```python
from build123d import *

# Parameters (mm, degrees)
F0_R     = 24.13
F1_DEPTH = 17.78
F2_R     = 39.733027
F2_R_2   = 24.13
F3_DEPTH = 25.4
F4_R     = 27.837104
F5_DEPTH = 19.05
F6_R     = 15.212569
F7_DEPTH = 12.7


with BuildPart() as f1:
    # F0 (on Top) → F1 (new body)
    with BuildSketch(Plane.XY):
        with Locations((-89.226432, 10.949461)):
            Circle(F0_R)
    extrude(amount=F1_DEPTH)

    # F2 (on face) → F3 (join)
    with BuildSketch(Plane.XY.offset(17.78)):
        with Locations((-89.226432, 10.949461)):
            Circle(F2_R)
        with Locations((-89.226432, 10.949461)):
            Circle(F2_R_2, mode=Mode.SUBTRACT)
        with Locations((-89.226432, 10.949461)):
            Circle(F2_R_2)
    extrude(amount=F3_DEPTH)

    # F4 (on face) → F5 (join)
    with BuildSketch(Plane.XY.offset(43.18)):
        with Locations((-89.226432, 10.949461)):
            Circle(F4_R)
    extrude(amount=F5_DEPTH)

    # F6 (on face) → F7 (join)
    with BuildSketch(Plane.XY.offset(62.23)):
        with Locations((-89.226432, 10.949461)):
            Circle(F6_R)
    extrude(amount=F7_DEPTH)


solid = f1.part
```
The model under review builds one solid part; all positions refer to its coordinate system, in mm. A direction names the side the tool comes from. Give positions to 0.01 mm unless a question says otherwise; leave off trailing zeros. Order: outer loops, then holes, each group sorted by start corner. A loop starts at its lowest first (then second) coordinate and runs counter-clockwise, first axis right, second up. Notation, with made-up numbers: (20, -7.5) - (36, -7.5) arc R16 ccw to (36, -0.5) - close; hole circle Ø2 at (75, 73). An arc over 180 degrees is marked (long way). Use CSV: the item, a comma, the result in double quotes. Start each with the question number.
Q1. We need section A-A, the plane x = -93. Write out the cut boundary in (y, z), and give its area (3 significant figures).
Q2. Clearance check with flat-ended pins moving along their axes: pin 1 Ø10 at (y, z) = (36.5, 51) entering from +X; pin 2 Ø1.5 at (x, y) = (-84, -8) entering from +Z; pin 3 Ø8 at (y, z) = (-9, 62.5) entering from +X. State where each tip first meets the part, or that it passes through.
Q3. Tool access review of faces 3 (the flat face through (-90, -15, 17.78)), 4 (the cylindrical face through (-74.716, 15.519, 68.491)), 5 (the cylindrical face through (-51.328, 22.884, 30.302)): name each direction out of +Z, -Z, +X, -X, +Y, -Y from which nothing blocks a thin tool from reaching the whole face with its end or side.
Q4. We need section C-C, the plane z = 66.5. Write out the cut boundary in (x, y).
Q5. To check wall thickness, follow line 1 along Z through (x, y) = (-90, -22); line 2 along Z through (x, y) = (-92, -7.5); line 3 along Y through (x, z) = (-88, 58). State the ranges of each line that lie inside material, in increasing order. Write a range as [from, to].
Q6. The part is to be moulded in two halves that separate along Y. For faces 1 (the flat face through (-89, 11, 74.93)), 2 (the cylindrical face through (-111.317, -5.989, 52.572)), say which applies: +Y half, -Y half, draft (parallel to the pull), parting line (faces both ways), or undercut.
Q7. We need section B-B, the plane y = 28. Write out the cut boundary in (x, z), and give its area (3 significant figures).
Q8. We need section D-D, the plane y = -6. Write out the cut boundary in (x, z).
Outcome:
1,outline,"(-28.6, 17.78) - (-12.88, 17.78) - (-12.88, 0) - (34.78, 0) - (34.78, 17.78) - (50.5, 17.78) - (50.5, 43.18) - (38.53, 43.18) - (38.53, 62.23) - (25.69, 62.23) - (25.69, 74.93) - (-3.79, 74.93) - (-3.79, 62.23) - (-16.63, 62.23) - (-16.63, 43.18) - (-28.6, 43.18) - close"
1,area,"4,280 mm^2"
2,pin 1,"stops at x = -70.45"
2,pin 2,"stops at z = 62.23"
2,pin 3,"stops at x = -66.42"
3,face 3,"-Z"
3,face 4,"+Z"
3,face 5,"+Z, -Z"
4,outline,"circle Ø30.43 at (-89.23, 10.95)"
5,line 1,"z = [17.78, 43.18]"
5,line 2,"z = [0, 62.23]"
5,line 3,"y = [-16.86, 38.76]"
6,face 1,"draft"
6,face 2,"parting line"
7,outline,"(-125.12, 17.78) - (-106.3, 17.78) - (-106.3, 0) - (-72.15, 0) - (-72.15, 17.78) - (-53.34, 17.78) - (-53.34, 43.18) - (-67.22, 43.18) - (-67.22, 62.23) - (-111.23, 62.23) - (-111.23, 43.18) - (-125.12, 43.18) - close"
7,area,"3,270 mm^2"
8,outline,"(-125.16, 17.78) - (-106.4, 17.78) - (-106.4, 0) - (-72.05, 0) - (-72.05, 17.78) - (-53.29, 17.78) - (-53.29, 43.18) - (-67.14, 43.18) - (-67.14, 62.23) - (-111.31, 62.23) - (-111.31, 43.18) - (-125.16, 43.18) - close"
